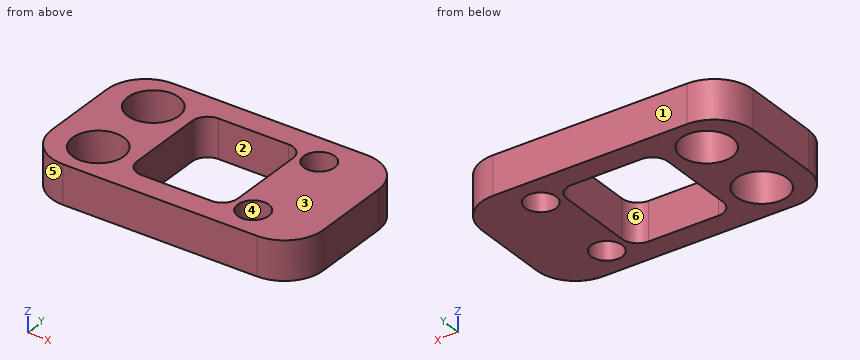
from build123d import *

# Parameters (mm, degrees)
ESQUISSE1_W             = 35
ESQUISSE1_H             = 20
BOSS_EXTRU_1_DEPTH      = 5
CONG_1_R                = 5
ESQUISSE7_R             = 2
ENL_V_MAT_EXTRU_2_DEPTH = 10
ESQUISSE6_R             = 3.3
ENL_V_MAT_EXTRU_3_DEPTH = 10
ESQUISSE9_W             = 13
ESQUISSE9_H             = 14
ENL_V_MAT_EXTRU_5_DEPTH = 10
CONG_2_R                = 2


with BuildPart() as part:
    # Esquisse1 → Boss.-Extru.1 (new body)
    with BuildSketch(Plane.XY):
        with Locations((-31.272929194, 23.850830526)):
            Rectangle(ESQUISSE1_W, ESQUISSE1_H)
    extrude(amount=BOSS_EXTRU_1_DEPTH)

    # Congé1
    cong_1_edges = [part.edges().sort_by_distance(p)[0] for p in [
        (-13.772929194, 13.850830526, 2.5),
        (-48.772929194, 13.850830526, 2.5),
        (-48.772929194, 33.850830526, 2.5),
        (-13.772929194, 33.850830526, 2.5),
    ]]
    fillet(cong_1_edges, radius=CONG_1_R)

    # Esquisse7 → Enlèv. mat.-Extru.2 (cut)
    with BuildSketch(Plane.XY.offset(5)):
        with Locations((-22.092006288, 29.850830526)):
            Circle(ESQUISSE7_R)
        with Locations((-22.092006288, 17.850830526)):
            Circle(ESQUISSE7_R)
    extrude(amount=-ENL_V_MAT_EXTRU_2_DEPTH, mode=Mode.SUBTRACT)

    # Esquisse6 → Enlèv. mat.-Extru.3 (cut)
    with BuildSketch(Plane.XY.offset(5)):
        with Locations((-42.772929194, 28.850830526)):
            Circle(ESQUISSE6_R)
        with Locations((-42.772929194, 18.850830526)):
            Circle(ESQUISSE6_R)
    extrude(amount=-ENL_V_MAT_EXTRU_3_DEPTH, mode=Mode.SUBTRACT)

    # Esquisse9 → Enlèv. mat.-Extru.5 (cut)
    with BuildSketch(Plane.XY.offset(5)):
        with Locations((-31.272929194, 23.850830526)):
            Rectangle(ESQUISSE9_W, ESQUISSE9_H)
    extrude(amount=-ENL_V_MAT_EXTRU_5_DEPTH, mode=Mode.SUBTRACT)

    # Congé2
    cong_2_edges = [part.edges().sort_by_distance(p)[0] for p in [
        (-24.772929194, 30.850830526, 2.5),
        (-24.772929194, 16.850830526, 2.5),
        (-37.772929194, 16.850830526, 2.5),
        (-37.772929194, 30.850830526, 2.5),
    ]]
    fillet(cong_2_edges, radius=CONG_2_R)


solid = part.part
Build history of the part. All positions in model axes, mm. Face numbers are marked on the shaded views. A direction names the side the tool comes from. Round coordinates to 2 decimals unless told otherwise and drop trailing zeros. Order: outer loops, then holes, each group sorted by start corner. A loop starts at its lowest first (then second) coordinate and runs counter-clockwise, first axis right, second up. Notation, with made-up numbers: M 22,74 L 29,74 A28 ccw 29,111 Z; hole C 75.5,65 d1. An arc over 180 degrees is marked long. Use CSV: the item, a comma, the result in double quotes. Start each with the question number.
(1) Cut at A-A on x = -32. List the corners of the cut face in (y, z).
(2) Drill centre lines: probe 1 along Y at (x, z) = (-28.5, 1.05); probe 2 along Y at (x, z) = (-42.5, 3.4); probe 3 along X at (y, z) = (20.25, 3.75). Where is each one in solid material? Low to high.
(3) Cut at B-B on y = 30.25. List the corners of the cut face in (x, z).
(4) Cut at D-D on x = -42. List the corners of the cut face in (y, z).
(5) Flat gauge pins, fed straight in: P1, Ø3, axis at y = 30.5, z = 4.5, coming from the +X side; P2, Ø6, axis at x = -42.77, y = 28.85, coming from the +Z side. Where does each tip first touch, or does it go through?
(6) Tool access for the marked faces 5 and 6: list every direction of +Z, -Z, +X, -X, +Y, -Y with a clear straight run to the whole face (end or side of a thin tool).
(7) Mould opens along Y. For the marked faces 1, 2, 3 and 4 say: +Y half, -Y half, draft (parallel to the pull), parting line (faces both ways), or undercut.
(8) Cut at C-C on y = 25. List the corners of the cut face in (x, z), then the cut area to 3 significant figures.
Findings:
1,outline,"M 13.85,0 L 16.85,0 L 16.85,5 L 13.85,5 Z; M 30.85,0 L 33.85,0 L 33.85,5 L 30.85,5 Z"
2,probe 1,"y = 13.85 to 16.85, 30.85 to 33.85"
2,probe 2,"y = 13.85 to 15.56, 22.14 to 25.56, 32.14 to 33.85"
2,probe 3,"x = -48.77 to -45.76, -39.78 to -37.77, -24.77 to -13.77"
3,outline,"M -48.57,0 L -45.76,0 L -45.76,5 L -48.57,5 Z; M -39.78,0 L -37.2,0 L -37.2,5 L -39.78,5 Z; M -25.34,0 L -24.05,0 L -24.05,5 L -25.34,5 Z; M -20.13,0 L -13.97,0 L -13.97,5 L -20.13,5 Z"
4,outline,"M 13.85,0 L 15.64,0 L 15.64,5 L 13.85,5 Z; M 22.06,0 L 25.64,0 L 25.64,5 L 22.06,5 Z; M 32.06,0 L 33.85,0 L 33.85,5 L 32.06,5 Z"
5,P1,"stops at x = -13.78"
5,P2,"passes through"
6,face 5,"+Z, -Z, -X, -Y"
6,face 6,"+Z, -Z"
7,face 1,"+Y half"
7,face 2,"undercut"
7,face 3,"draft"
7,face 4,"undercut"
8,outline,"M -48.77,0 L -37.77,0 L -37.77,5 L -48.77,5 Z; M -24.77,0 L -13.77,0 L -13.77,5 L -24.77,5 Z"
8,area,"110 mm^2"
